from build123d import *

# Parameters (mm, degrees)
F1_DEPTH = 1.016
F0_R     = 6.604
F0_R_2   = 11.590192
F0_R_3   = 6.096
F0_R_4   = 4.572
F2_DEPTH = 1.016


with BuildPart() as f1:
    # F0 (on Front) → F1 (new body)
    with BuildSketch(Plane.XZ):
        with BuildLine():
            ThreePointArc((71.748899, -48.69655), (82.234953, -44.90898), (87.880266, -35.294748))
            Line((87.880266, -35.294748), (97.438355, 29.049238))
            ThreePointArc((97.438355, 29.049238), (96.779702, 32.50332), (94.114392, 34.796925))
            ThreePointArc((94.114392, 34.796925), (8.063382, 56.200754), (-80.144331, 65.272659))
            ThreePointArc((-80.144331, 65.272659), (-85.435827, 62.950768), (-88.040151, 57.792414))
            Line((-88.040151, 57.792414), (-100.186102, -40.73111))
            ThreePointArc((-100.186102, -40.73111), (-98.290515, -46.492526), (-92.639901, -48.69655))
            Line((-92.639901, -48.69655), (71.748899, -48.69655))
        make_face()
        with BuildLine():
            ThreePointArc((-68.658263, 50.559288), (4.937485, 42.307161), (77.003889, 25.252396))
            ThreePointArc((77.003889, 25.252396), (80.533579, 22.574015), (81.452525, 18.239506))
            Line((81.452525, 18.239506), (74.024657, -31.764068))
            ThreePointArc((74.024657, -31.764068), (72.957694, -33.701903), (70.884118, -34.472551))
            Line((70.884118, -34.472551), (33.536372, -34.472551))
            ThreePointArc((33.536372, -34.472551), (31.558624, -34.788397), (29.77762, -35.704516))
            ThreePointArc((29.77762, -35.704516), (11.863571, -41.576006), (-6.050479, -35.704516))
            ThreePointArc((-6.050479, -35.704516), (-7.831482, -34.788397), (-9.80923, -34.472551))
            Line((-9.80923, -34.472551), (-81.49242, -34.472551))
            ThreePointArc((-81.49242, -34.472551), (-83.870868, -33.40079), (-84.643565, -30.909079))
            Line((-84.643565, -30.909079), (-75.286183, 44.994587))
            ThreePointArc((-75.286183, 44.994587), (-73.066979, 49.080863), (-68.658263, 50.559288))
        make_face(mode=Mode.SUBTRACT)
    extrude(amount=F1_DEPTH)

    # F0 (on Front) → F2 (join)
    with BuildSketch(Plane.XZ):
        with BuildLine():
            ThreePointArc((81.452525, 18.239506), (80.533579, 22.574015), (77.003889, 25.252396))
            ThreePointArc((77.003889, 25.252396), (4.937485, 42.307161), (-68.658263, 50.559288))
            ThreePointArc((-68.658263, 50.559288), (-73.066979, 49.080863), (-75.286183, 44.994587))
            Line((-75.286183, 44.994587), (-84.643565, -30.909079))
            ThreePointArc((-84.643565, -30.909079), (-83.870868, -33.40079), (-81.49242, -34.472551))
            Line((-81.49242, -34.472551), (-9.80923, -34.472551))
            ThreePointArc((-9.80923, -34.472551), (-7.831482, -34.788397), (-6.050479, -35.704516))
            ThreePointArc((-6.050479, -35.704516), (11.863571, -41.576006), (29.77762, -35.704516))
            ThreePointArc((29.77762, -35.704516), (31.558624, -34.788397), (33.536372, -34.472551))
            Line((33.536372, -34.472551), (70.884118, -34.472551))
            ThreePointArc((70.884118, -34.472551), (72.957694, -33.701903), (74.024657, -31.764068))
            Line((74.024657, -31.764068), (81.452525, 18.239506))
        make_face()
        with Locations((-28.321732, -27.52208)):
            Circle(F0_R, mode=Mode.SUBTRACT)
        with Locations((11.999482, -11.534391)):
            Circle(F0_R_2, mode=Mode.SUBTRACT)
        with Locations((38.945176, -17.489335)):
            Circle(F0_R, mode=Mode.SUBTRACT)
        with Locations((11.999482, -11.534391)):
            Circle(F0_R_2)
        with Locations((11.999482, -11.534391)):
            Circle(F0_R_3, mode=Mode.SUBTRACT)
        with Locations((11.999482, -11.534391)):
            Circle(F0_R_3)
        with Locations((11.999482, -11.534391)):
            Circle(F0_R_4, mode=Mode.SUBTRACT)
    extrude(amount=F2_DEPTH)


solid = f1.part
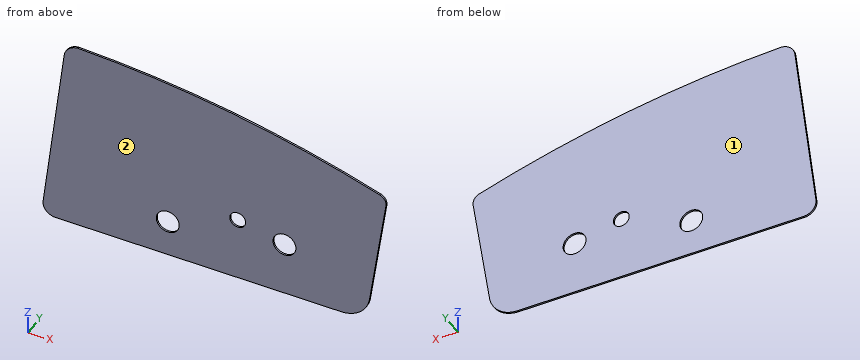
The listing builds one solid part. Answer for the finished solid, in the listing's coordinates (mm). Face numbers are marked on the shaded views. Give positions to 0.01 mm unless a question says otherwise; leave off trailing zeros. Write each loop counter-clockwise with the first axis right and the second up, starting at its lowest first coordinate (ties: lowest second). Pieces come first, ordered by that corner, then holes.
1) Find the intervals of material crossed by L1, parallel to X at y = -0.15, z = -12; L2, parallel to Z at x = -23.5, y = -0.1; L3, parallel to X at y = -0.25, z = -19.5, in increasing order.
2) Section B-B (y = -0.85) is taken. Write down the section's boundary in (x, z).
3) For a pull along Y with two mould halves and no side action, classify the marked faces 1 and 2 as pulls with the +Y half, pulls with the -Y half, needs draft (parallel to the pull), parting line crosses it, or undercut.
4) Section A-A (x = 42) is taken. Write down the section's boundary in (y, z), and give its area (3 significant figures).
5) Section C-C (z = 18) is taken. Write down the section's boundary in (x, y).
6) Section D-D (x = 78) is taken. Write down the section's boundary in (y, z), and give its area (3 significant figures).
Response:
1. L1: x = -96.64 to 7.45, 16.55 to 35.27, 42.62 to 91.34
1. L2: z = -48.7 to -32.03, -23.01 to 60.9
1. L3: x = -97.57 to 32.65, 45.24 to 90.23
2. outline: (-100.19, -40.73) arc R7.11 ccw to (-92.64, -48.7) - (71.75, -48.7) arc R16.41 ccw to (87.88, -35.29) - (97.44, 29.05) arc R5.33 ccw to (94.11, 34.8) arc R628.07 ccw to (-80.14, 65.27) arc R8.55 ccw to (-88.04, 57.79) - close; hole circle Ø13.21 at (-28.32, -27.52); hole circle Ø9.14 at (12, -11.53); hole circle Ø13.21 at (38.95, -17.49)
3. face 1: pulls with the +Y half
3. face 2: pulls with the -Y half
4. outline: (-1.02, -48.7) - (0, -48.7) - (0, -23.34) - (-1.02, -23.34) - close; (-1.02, -11.63) - (0, -11.63) - (0, 49.3) - (-1.02, 49.3) - close
4. area: 87.7 mm2
5. outline: (-92.95, -1.02) - (95.8, -1.02) - (95.8, 0) - (-92.95, 0) - close
6. outline: (-1.02, -47.46) - (0, -47.46) - (0, 39.8) - (-1.02, 39.8) - close
6. area: 88.7 mm2
